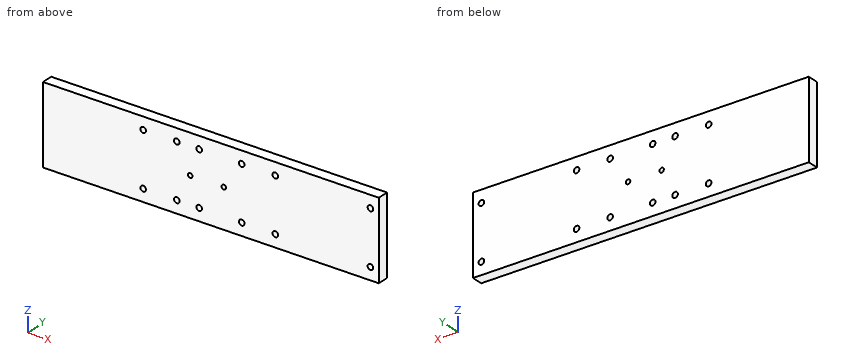
from build123d import *

# Parameters (mm, degrees)
F0_W     = 300
F0_H     = 70
F0_R     = 2.5
F0_R_2   = 2
F1_DEPTH = 10


with BuildPart() as f1:
    # F0 (on Front) → F1 (new body)
    with BuildSketch(Plane.XZ):
        with Locations((30.5, 16.277353)):
            Rectangle(F0_W, F0_H)
        with Locations((-30, -7.722647)):
            Circle(F0_R, mode=Mode.SUBTRACT)
        with Locations((0, -7.722647)):
            Circle(F0_R, mode=Mode.SUBTRACT)
        with Locations((20, -7.722647)):
            Circle(F0_R, mode=Mode.SUBTRACT)
        with Locations((58, -7.722647)):
            Circle(F0_R, mode=Mode.SUBTRACT)
        with Locations((88, -7.722647)):
            Circle(F0_R, mode=Mode.SUBTRACT)
        with Locations((173, -7.722647)):
            Circle(F0_R, mode=Mode.SUBTRACT)
        with Locations((12, 16.277353)):
            Circle(F0_R_2, mode=Mode.SUBTRACT)
        with Locations((-30, 40.277353)):
            Circle(F0_R, mode=Mode.SUBTRACT)
        with Locations((0, 40.277353)):
            Circle(F0_R, mode=Mode.SUBTRACT)
        with Locations((20, 40.277353)):
            Circle(F0_R, mode=Mode.SUBTRACT)
        with Locations((42, 16.277353)):
            Circle(F0_R_2, mode=Mode.SUBTRACT)
        with Locations((58, 40.277353)):
            Circle(F0_R, mode=Mode.SUBTRACT)
        with Locations((88, 40.277353)):
            Circle(F0_R, mode=Mode.SUBTRACT)
        with Locations((173, 40.277353)):
            Circle(F0_R, mode=Mode.SUBTRACT)
    extrude(amount=F1_DEPTH)


solid = f1.part
The listing builds one solid part. Answer for the finished solid, in the listing's coordinates (mm). Give positions to 0.01 mm unless a question says otherwise; leave off trailing zeros. Order: outer loops, then holes, each group sorted by start corner. A loop starts at its lowest first (then second) coordinate and runs counter-clockwise, first axis right, second up. Notation, with made-up numbers: (-11, 1.5) -> (1, 1.5) arc R32 ccw to (1, 28.5) -> close; hole circle Ø2 at (63.5, -24.75). An arc over 180 degrees is marked (long way). Put each result on its own line as item: value.
Item 1: Given P1, Ø4.5, axis at x = 58, z = 40.28, coming from the -Y side, flat-ended and moving along its own axis, determine where the tip first touches the part or whether it passes through.
Established:
P1: passes through
Item 2: Straight lines are drawn through the part: line 1 (X direction, y = -9, z = 14.5); line 2 (Z direction, x = 86.5, y = -5); line 3 (Z direction, x = 60, y = -2.25). For each, find the intervals that lie inside material, in ascending order.
Established:
line 1: x = -119.5 to 11.08, 12.92 to 41.08, 42.92 to 180.5
line 2: z = -18.72 to -9.72, -5.72 to 38.28, 42.28 to 51.28
line 3: z = -18.72 to -9.22, -6.22 to 38.78, 41.78 to 51.28
Item 3: A cutting plane is placed at A-A on x = 173. Give the vertices of the cut face in (y, z), plus the area to 3 significant figures.
Established:
outline: (-10, -18.72) -> (0, -18.72) -> (0, -10.22) -> (-10, -10.22) -> close; (-10, -5.22) -> (0, -5.22) -> (0, 37.78) -> (-10, 37.78) -> close; (-10, 42.78) -> (0, 42.78) -> (0, 51.28) -> (-10, 51.28) -> close
area: 600 mm^2
